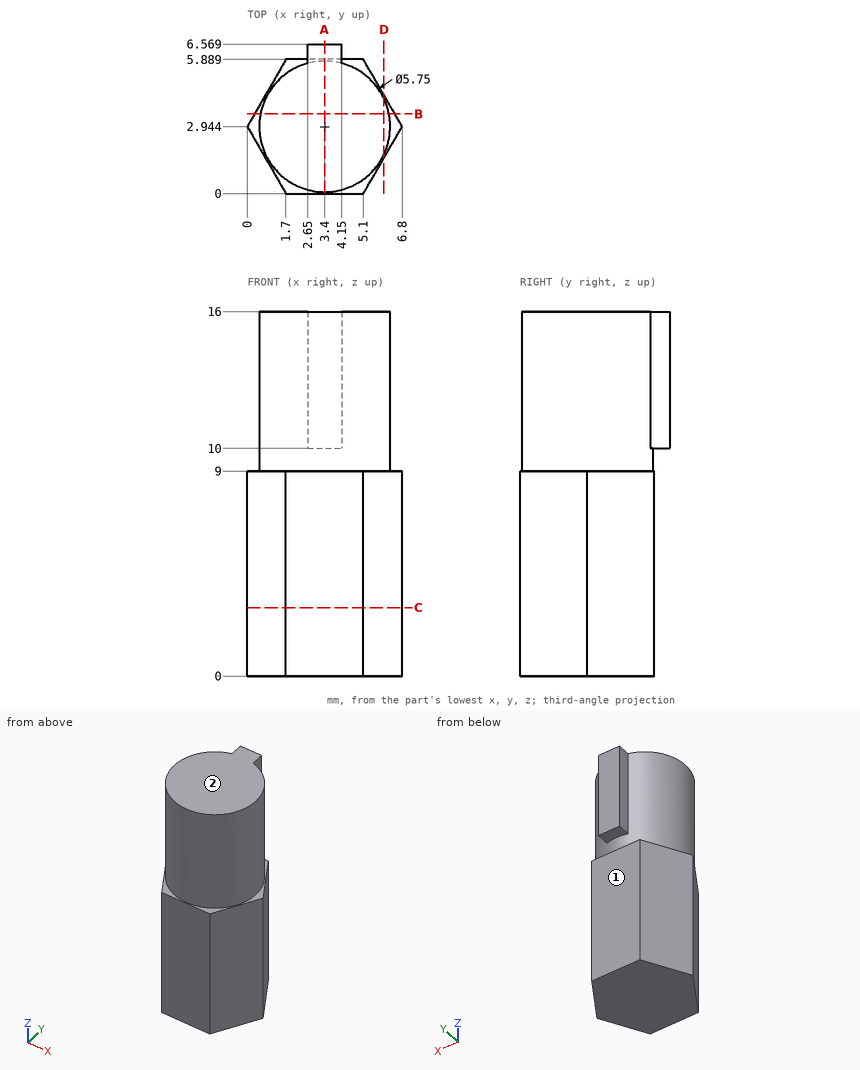
Here's the drawing with two shaded views (mm, measured from the low corner). I have some questions. A direction names the side the tool comes from. Coordinates: 2 decimals unless noted, no trailing zeros. Write each loop counter-clockwise with the first axis right and the second up, starting at its lowest first coordinate (ties: lowest second). Pieces come first, ordered by that corner, then holes.
Item 1: I want a section at B-B on y = 3.5. Write out the boundary of the cut face in (x, z).
Item 2: I want a section at A-A on x = 3.4. Write out the boundary of the cut face in (y, z).
Item 3: On a 3-axis mill with a long thin cutter (end or side, diameter ignored), from which of +Z, -Z, +X, -X, +Y, -Y can I reach the whole of each face in a straight line? I mean the marked faces 1 and 2. Say none if no direction works.
Item 4: Will these pins go through, and if not, where does the flat tip stop? pin 1 (2 mm diameter, centred on y = 5.5, z = 6.5, fed in from -X); pin 2 (2.5 mm diameter, centred on x = 3, z = 4, fed in from +Y).
Item 5: If I drill on line 1 (Z direction, x = 0.5, y = 3.5); line 2 (Y direction, x = 3.25, z = 5.75); line 3 (Y direction, x = 4.5, z = 12.5), over which ranges is the centre line in solid material (lowest first)?
Item 6: I want a section at C-C on z = 3. Write out the boundary of the cut face in (x, y) (1 decimal).
Item 7: I want a section at D-D on x = 6. Write out the boundary of the cut face in (y, z).
Findings below:
1. outline: (0.32, 0) - (6.48, 0) - (6.48, 9) - (6.22, 9) - (6.22, 16) - (0.58, 16) - (0.58, 9) - (0.32, 9) - close
2. outline: (0, 0) - (5.89, 0) - (5.89, 9) - (5.82, 9) - (5.82, 10) - (6.57, 10) - (6.57, 16) - (0.07, 16) - (0.07, 9) - (0, 9) - close
3. face 1: -Z, +X, -X, +Y
3. face 2: +Z, +X, -X, +Y, -Y
4. pin 1: stops at x = 0.9
4. pin 2: stops at y = 5.89
5. line 1: z = 0 to 9
5. line 2: y = 0 to 5.89
5. line 3: y = 0.29 to 5.6
6. outline: (0, 2.9) - (1.7, 0) - (5.1, 0) - (6.8, 2.9) - (5.1, 5.9) - (1.7, 5.9) - close
7. outline: (1.56, 0) - (4.33, 0) - (4.33, 9) - (4.17, 9) - (4.17, 16) - (1.72, 16) - (1.72, 9) - (1.56, 9) - close
